The model under review builds one solid part; all positions refer to its coordinate system, in mm. Face numbers are marked on the shaded views. Coordinates: 2 decimals unless noted, no trailing zeros. Order: outer loops, then holes, each group sorted by start corner. A loop starts at its lowest first (then second) coordinate and runs counter-clockwise, first axis right, second up. Notation, with made-up numbers: (-30.5, -10.75) - (8.5, -10.75) arc R14 cw to (8.5, -0.75) - close; hole circle Ø7 at (34, 13). An arc over 180 degrees is marked (long way). Answer in a Markdown table with one row per item.
```python
from build123d import *

# Parameters (mm, degrees)
F0_R     = 3.175
F1_DEPTH = 25.4
F2_SIZE  = 0.508
F3_R     = 1.5875
F4_DEPTH = 3.175


with BuildPart() as f1:
    # F0 (on Front) → F1 (new body)
    with BuildSketch(Plane.XZ):
        Circle(F0_R)
    extrude(amount=F1_DEPTH)

    # F2
    f2_edges = [f1.edges().sort_by_distance(p)[0] for p in [
        (-3.175, -25.4, 0),
    ]]
    chamfer(f2_edges, length=F2_SIZE)

    # F3 (on Right) → F4 (cut, symmetric)
    with BuildSketch(Plane.YZ):
        with Locations((-3.175, 0)):
            Circle(F3_R)
    extrude(amount=F4_DEPTH, both=True, mode=Mode.SUBTRACT)


solid = f1.part
```
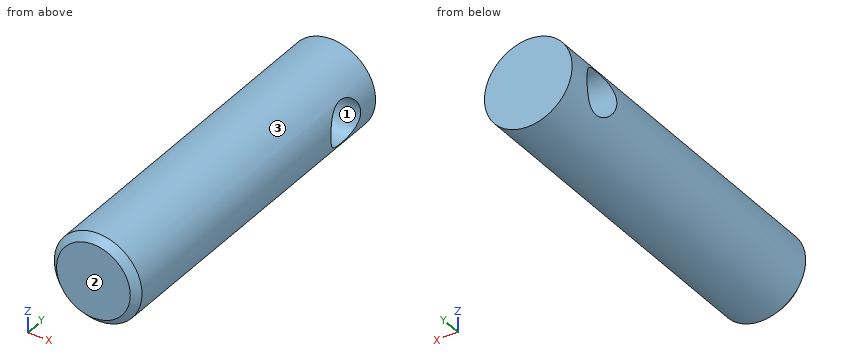
Item 1: Clearance check with flat-ended pins moving along their axes: pin 1 Ø1.5 at (y, z) = (-21, -0.5) entering from -X (3 decimals); pin 2 Ø2 at (x, y) = (-1.5, -8.5) entering from +Z; pin 3 Ø2 at (x, y) = (2, -22) entering from +Z. State where each tip first meets the part, or that it passes through.
Check values:
| item | result |
|---|---|
| pin 1 | x = -3.175 |
| pin 2 | z = 3.14 |
| pin 3 | z = 3.01 |
Item 2: We need section B-B, the plane x = 0. Write out the cut boundary in (y, z) (1 decimal).
Check values:
| item | result |
|---|---|
| outline | (-25.4, -2.7) - (-24.9, -3.2) - (0, -3.2) - (0, 3.2) - (-24.9, 3.2) - (-25.4, 2.7) - close; hole circle Ø3.2 at (-3.2, 0) |
Item 3: Mouldability with a two-part tool opening along Z and no side actions: class the marked faces 1, 2 and 3 as +Z half, -Z half, draft (parallel to the pull), parting line (faces both ways), or undercut.
Check values:
| item | result |
|---|---|
| face 1 | undercut |
| face 2 | draft |
| face 3 | parting line |
Item 4: To check wall thickness, follow line 1 (Y direction, x = 1.5, z = 0); line 2 (Y direction, x = 2.25, z = 1); line 3 (X direction, y = -22.5, z = 2.75). State the ranges of each line that lie inside material, in increasing order. Write a range as from..to.
Check values:
| item | result |
|---|---|
| line 1 | -25.4..-4.76, -1.59..0 |
| line 2 | -25.4..-4.41, -1.94..0 |
| line 3 | -1.59..1.59 |
Item 5: We need section C-C, the plane y = -8.5. Write out the cut boundary in (x, z) (3 decimals), then the cut area to 3 significant figures.
Check values:
| item | result |
|---|---|
| outline | circle Ø6.35 at (0, 0) |
| area | 31.7 mm^2 |
Item 6: We need section A-A, the plane z = 0. Write out the cut boundary in (x, y) (1 decimal), then the cut area to 3 significant figures.
Check values:
| item | result |
|---|---|
| outline | (-3.2, -24.9) - (-2.7, -25.4) - (2.7, -25.4) - (3.2, -24.9) - (3.2, -4.8) - (-3.2, -4.8) - close; (-3.2, -1.6) - (3.2, -1.6) - (3.2, 0) - (-3.2, 0) - close |
| area | 141 mm^2 |
